The drawing under review shows one solid part. Ordinate dimensions are in mm from its lowest x, y, z. A direction names the side the tool comes from. Give positions to 0.01 mm unless a question says otherwise; leave off trailing zeros. Order: outer loops, then holes, each group sorted by start corner. A loop starts at its lowest first (then second) coordinate and runs counter-clockwise, first axis right, second up. Notation, with made-up numbers: (-19.75, 88.5) - (-2.75, 88.5) arc R15 ccw to (-2.75, 95.5) - close; hole circle Ø6 at (36.25, -19). An arc over 180 degrees is marked (long way). Answer as a JSON object with one key per item and string values. Group by question number.
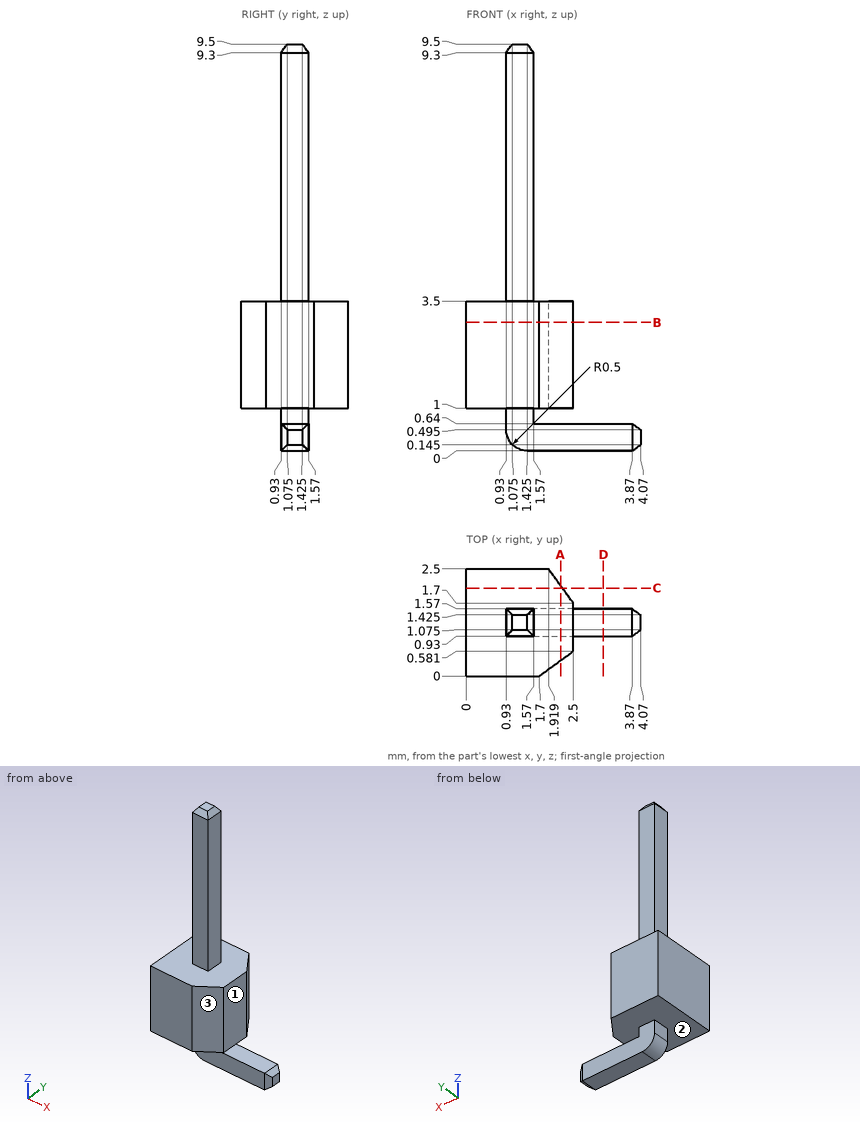
1) For the marked faces 1, 2 and 3, list the 3-axis set-ups (+Z, -Z, +X, -X, +Y, -Y) from which the entire face can be reached by the end or side of a thin tool; tool diameter is ignored.
2) For pin 1 (0.5 mm diameter, centred on x = 2.5, y = 1.5, fed in from +Z); pin 2 (0.7 mm diameter, centred on y = 1, z = 5.5, fed in from +X); pin 3 (0.7 mm diameter, centred on y = 1.5, z = 5.5, fed in from -X), all flat-tipped, find the tip position at first contact; note any pin that passes through.
3) For line 1 (Z direction, x = 1.6, y = 1.15); line 2 (Y direction, x = 1.3, z = 7.5); line 3 (Z direction, x = 1.65, y = 0.6), list the stretches that pass through material, from the lowest coordinate up.
4) Consider section B-B (z = 3). Give the boundary of the cut face in (x, y).
5) Consider section A-A (x = 2.2). Give the boundary of the cut face in (y, z).
6) Consider section D-D (x = 3.2). Give the boundary of the cut face in (y, z).
7) Consider section C-C (y = 2.05). Give the boundary of the cut face in (x, z).
Result set:
{
 "1": {"face 1": "+Z, +X, +Y, -Y", "face 2": "none", "face 3": "+Z, -Z, +X, -Y"},
 "2": {"pin 1": "stops at z = 3.5", "pin 2": "stops at x = 1.57", "pin 3": "stops at x = 0.93"},
 "3": {"line 1": "z = 0 to 0.64, 1 to 3.5", "line 2": "y = 0.93 to 1.57", "line 3": "z = 1 to 3.5"},
 "4": {"outline": "(0, 0) - (1.7, 0) - (2.5, 0.58) - (2.5, 1.7) - (1.92, 2.5) - (0, 2.5) - close"},
 "5": {"outline": "(0.36, 1) - (2.11, 1) - (2.11, 3.5) - (0.36, 3.5) - close; (0.93, 0) - (1.57, 0) - (1.57, 0.64) - (0.93, 0.64) - close"},
 "6": {"outline": "(0.93, 0) - (1.57, 0) - (1.57, 0.64) - (0.93, 0.64) - close"},
 "7": {"outline": "(0, 1) - (2.25, 1) - (2.25, 3.5) - (0, 3.5) - close"}
}
